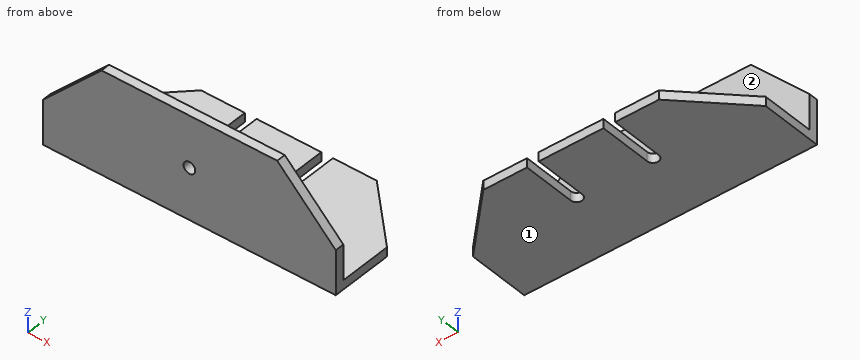
```python
from build123d import *

# Parameters (mm, degrees)
EXTRUDE_THIN1_DEPTH = 100
CUT_EXTRUDE1_DEPTH  = 36.197996578
CHAMFER1_SIZE       = 20
CHAMFER2_SIZE       = 20
SKETCH3_R           = 2
CUT_EXTRUDE2_DEPTH  = 42.225


with BuildPart() as part:
    # Sketch1 → Extrude-Thin1 (new body)
    with BuildSketch(Plane(origin=(0, 0, 0), x_dir=(0, 0, -1), z_dir=(1, 0, 0))):
        Polygon((0, 0), (32.072996578, 0), (32.072996578, 38.1), (35.197996578, 38.1), (35.197996578, -3.125), (0, -3.125), align=None)
    extrude(amount=EXTRUDE_THIN1_DEPTH)

    # Sketch2 → Cut-Extrude1 (cut, through all)
    with BuildSketch(Plane(origin=(0, 0, -35.197996578), x_dir=(-1, 0, 0), z_dir=(0, 0, -1))):
        with BuildLine():
            Line((-61.05, 20), (-61.05, 38.1))
            Line((-61.05, 38.1), (-65.05, 38.1))
            Line((-65.05, 38.1), (-65.05, 20))
            ThreePointArc((-65.05, 20), (-63.05, 18), (-61.05, 20))
        make_face()
        with BuildLine():
            Line((-38.95, 20), (-38.95, 38.1))
            Line((-38.95, 38.1), (-34.95, 38.1))
            Line((-34.95, 38.1), (-34.95, 20))
            ThreePointArc((-34.95, 20), (-36.95, 18), (-38.95, 20))
        make_face()
    extrude(amount=-CUT_EXTRUDE1_DEPTH, mode=Mode.SUBTRACT)

    # Chamfer1
    chamfer1_edges = [part.edges().sort_by_distance(p)[0] for p in [
        (0, 38.1, -33.635496578),
        (100, 38.1, -33.635496578),
    ]]
    chamfer(chamfer1_edges, length=CHAMFER1_SIZE)

    # Chamfer2
    chamfer2_edges = [part.edges().sort_by_distance(p)[0] for p in [
        (100, -1.5625, 0),
        (0, -1.5625, 0),
    ]]
    chamfer(chamfer2_edges, length=CHAMFER2_SIZE)

    # Sketch3 → Cut-Extrude2 (cut, through all)
    with BuildSketch(Plane.XZ.offset(3.125)):
        with Locations(Location((50, -17.598998289, 0), (0, 0, 270))):  # turned: the seam where the file's is
            Circle(SKETCH3_R)
    extrude(amount=-CUT_EXTRUDE2_DEPTH, mode=Mode.SUBTRACT)


solid = part.part
```
Check sheet for the modelled part. Datum: model origin and axes. Units: mm. Face numbers are marked on the shaded views. A direction names the side the tool comes from. Round coordinates to 2 decimals unless told otherwise and drop trailing zeros. Order: outer loops, then holes, each group sorted by start corner. A loop starts at its lowest first (then second) coordinate and runs counter-clockwise, first axis right, second up. Notation, with made-up numbers: M 17.5,9 L 72.5,9 A24 ccw 72.5,48 Z; hole C 52,-30.5 d9. An arc over 180 degrees is marked long. Answer in a Markdown table with one row per item.
(1) Section check B-B on y = 22. Record the boundary of the cut face in (x, z).
Findings:
| item | result |
|---|---|
| outline | M 3.9,-35.2 L 34.95,-35.2 L 34.95,-32.07 L 3.9,-32.07 Z; M 38.95,-35.2 L 61.05,-35.2 L 61.05,-32.07 L 38.95,-32.07 Z; M 65.05,-35.2 L 96.1,-35.2 L 96.1,-32.07 L 65.05,-32.07 Z |
(2) Section check D-D on y = 35. Record the boundary of the cut face in (x, z), plus the area to 3 significant figures.
Findings:
| item | result |
|---|---|
| outline | M 16.9,-35.2 L 34.95,-35.2 L 34.95,-32.07 L 16.9,-32.07 Z; M 38.95,-35.2 L 61.05,-35.2 L 61.05,-32.07 L 38.95,-32.07 Z; M 65.05,-35.2 L 83.1,-35.2 L 83.1,-32.07 L 65.05,-32.07 Z |
| area | 182 mm^2 |
(3) Material ranges on line 1 along X through (y, z) = (32.5, -32.5); line 2 along Y through (x, z) = (92.5, -20) (3 decimals); line 3 along Z through (x, y) = (28, 1), recorded low to high. Write a range as from..to.
Findings:
| item | result |
|---|---|
| line 1 | x = 14.4..34.95, 38.95..61.05, 65.05..85.6 |
| line 2 | y = -3.125..0 |
| line 3 | z = -35.2..-32.07 |
(4) Section check C-C on x = 84.5. Record the boundary of the cut face in (y, z) (3 decimals).
Findings:
| item | result |
|---|---|
| outline | M -3.125,-35.198 L 33.6,-35.198 L 33.6,-32.073 L 0,-32.073 L 0,-4.5 L -3.125,-4.5 Z |
(5) Section check A-A on x = 50. Record the boundary of the cut face in (y, z) (3 decimals).
Findings:
| item | result |
|---|---|
| outline | M -3.125,-35.198 L 38.1,-35.198 L 38.1,-32.073 L 0,-32.073 L 0,-19.599 L -3.125,-19.599 Z; M -3.125,-15.599 L 0,-15.599 L 0,0 L -3.125,0 Z |
(6) Gauge pin test, flat ends, axial feed: pin 1 (3 mm diameter, centred on x = 81.5, z = -9.5, fed in from +Y); pin 2 (10 mm diameter, centred on x = 34.5, y = 11.5, fed in from +Z); pin 3 (3.5 mm diameter, centred on y = 29.5, z = -33, fed in from -X). Record the tip position at first contact, or that the pin passes through.
Findings:
| item | result |
|---|---|
| pin 1 | stops at y = 0 |
| pin 2 | stops at z = -32.07 |
| pin 3 | stops at x = 9.65 |
(7) Set-up check for the marked faces 1 and 2: record each of +Z, -Z, +X, -X, +Y, -Y from which the full face is reachable in a straight line by a thin tool's end or side.
Findings:
| item | result |
|---|---|
| face 1 | -Z, +X, -X, +Y, -Y |
| face 2 | +Z, +X, -X, +Y |
